Autodesk Inventor part; units mm, degrees
ref_plane "YZ Plane" through (0, 0, 0) normal (1, 0, 0) x (0, 1, 0)
ref_plane "XZ Plane" through (0, 0, 0) normal (0, 1, 0) x (-1, 0, 0)
ref_plane "XY Plane" through (0, 0, 0) normal (0, 0, 1) x (1, 0, 0)
sketch "Sketch1" plane through (0, 0, 0) normal (0, 0, 1) x (1, 0, 0)
  line L0 (-45, -34) -> (45, -34)
  line L1 (52, -27) -> (52, 27)
  line L2 (45, 34) -> (-45, 34)
  line L3 (-52, 27) -> (-52, -27)
  line L4 (-52, -34) -> (52, 34) construction
  line L5 (52, -34) -> (-52, 34) construction
  line L6 (-45, 27) -> (45, 27) construction
  line L7 (45, 27) -> (45, -27) construction
  line L8 (45, -27) -> (-45, -27) construction
  line L9 (-45, -27) -> (-45, 27) construction
  arc A0 (-45, 34) -> (-52, 27) centre (-45, 27) ccw
  arc A1 (52, 27) -> (45, 34) centre (45, 27) ccw
  arc A2 (45, -34) -> (52, -27) centre (45, -27) ccw
  arc A3 (-52, -27) -> (-45, -34) centre (-45, -27) ccw
  point P0 (0, 0)
  dimension "d0" = 104
  dimension "d1" = 68
  dimension "d2" = 54
  dimension "d3" = 90
extrude "Extrusion1" add sketch "Sketch1" along normal mid plane 4
sketch "Sketch2" plane through (0, 0, 2) normal (0, 0, 1) x (1, 0, 0)
  line L0 (45, 34) -> (-45, 34)
  arc A0 (-45, 34) -> (-52, 27) centre (-45, 27) ccw
  line L1 (-52, 27) -> (-52, -27)
  arc A1 (-52, -27) -> (-45, -34) centre (-45, -27) ccw
  line L2 (-45, -34) -> (45, -34)
  arc A2 (45, -34) -> (52, -27) centre (45, -27) ccw
  line L3 (52, -27) -> (52, 27)
  arc A3 (52, 27) -> (45, 34) centre (45, 27) ccw
  circle A4 centre (-45, 27) radius 2.75
  circle A5 centre (45, 27) radius 2.75
  circle A6 centre (45, -27) radius 2.75
  circle A7 centre (-45, -27) radius 2.75
  point P0 (0, 0)
  dimension "d7" = 5.5
extrude "Extrusion2" add sketch "Sketch2" along normal blind 5.3 contours A4 | A5 | A6 | A7
sketch "Sketch3" plane through (0, 0, -2) normal (0, 0, -1) x (-1, 0, 0)
  line L0 (45, 34) -> (-45, 34)
  arc A0 (-45, 34) -> (-52, 27) centre (-45, 27) ccw
  line L1 (-52, 27) -> (-52, -27)
  arc A1 (-52, -27) -> (-45, -34) centre (-45, -27) ccw
  line L2 (-45, -34) -> (45, -34)
  arc A2 (45, -34) -> (52, -27) centre (45, -27) ccw
  line L3 (52, -27) -> (52, 27)
  arc A3 (52, 27) -> (45, 34) centre (45, 27) ccw
  circle A4 centre (-45, 27) radius 2.75
  point P0 (0, 0)
hole "Hole1" at (-45, -27, -2) at (45, -27, -2) at (45, 27, -2) at (-45, 27, -2) direction (0, 0, 1) diameter 2.642 end through all
sketch "Sketch4" plane through (0, 0, 2) normal (0, 0, 1) x (1, 0, 0)
  line L0 (-12.5, -12.5) -> (12.5, -12.5)
  line L1 (12.5, -12.5) -> (12.5, 12.5)
  line L2 (12.5, 12.5) -> (-12.5, 12.5)
  line L3 (-12.5, 12.5) -> (-12.5, -12.5)
  line L4 (-12.5, -12.5) -> (12.5, 12.5) construction
  line L5 (12.5, -12.5) -> (-12.5, 12.5) construction
  point P0 (0, 0)
  dimension "d17" = 25
extrude "Extrusion3" cut sketch "Sketch4" against normal blind 3.35
properties part number "BackBracket" material "Steel, Mild"
Can you work these out from the model? Positions are in its coordinate system, mm. A direction names the side the tool comes from. Round coordinates to 2 decimals unless told otherwise and drop trailing zeros. Write each loop counter-clockwise with the first axis right and the second up, starting at its lowest first coordinate (ties: lowest second). Pieces come first, ordered by that corner, then holes. Notation, with made-up numbers: M -35,-16.75 L 2,-16.75 A15 ccw 2,-3.75 Z; hole C -21,80.25 d9. An arc over 180 degrees is marked long. Use a Markdown table: item, result.
Item 1: For pin 1 Ø20.5 at (x, y) = (-4.5, -4.5) entering from +Z; pin 2 Ø4 at (x, y) = (-45, -27) entering from +Z; pin 3 Ø5 at (y, z) = (-24.5, 6) entering from +X; pin 4 Ø5 at (x, z) = (40, 5.5) entering from +Y, each with a flat end and sliding along its axis, tell me the tip position at first contact or that it passes through.
Found:
| item | result |
|---|---|
| pin 1 | stops at z = 2 |
| pin 2 | stops at z = 7.3 |
| pin 3 | stops at x = 47.75 |
| pin 4 | stops at y = 28.15 |
Item 2: I want a section at A-A (y = -4.5). List the corners of the cut face in (x, z) for me, and give its area (3 significant figures).
Found:
| item | result |
|---|---|
| outline | M -52,-2 L 52,-2 L 52,2 L 12.5,2 L 12.5,-1.35 L -12.5,-1.35 L -12.5,2 L -52,2 Z |
| area | 332 mm2 |
Item 3: I want a section at C-C (x = 25.5). List the corners of the cut face in (y, z) for me.
Found:
| item | result |
|---|---|
| outline | M -34,-2 L 34,-2 L 34,2 L -34,2 Z |
Item 4: I want a section at B-B (x = -8). List the corners of the cut face in (y, z) for me, and give its area (3 significant figures).
Found:
| item | result |
|---|---|
| outline | M -34,-2 L 34,-2 L 34,2 L 12.5,2 L 12.5,-1.35 L -12.5,-1.35 L -12.5,2 L -34,2 Z |
| area | 188 mm2 |
Item 5: Which directions (+Z, -Z, +X, -X, +Y, -Y) give clear straight access to the entire face, cutting with the end or side of a thin tool? Please do faces 1 (the face through (12.5, 0, 0)), 2 (the face through (46.17, -26.39, 2.72)).
Found:
| item | result |
|---|---|
| face 1 | +Z |
| face 2 | +Z, -Z |
Item 6: I want a section at D-D (y = 14). List the corners of the cut face in (x, z) for me.
Found:
| item | result |
|---|---|
| outline | M -52,-2 L 52,-2 L 52,2 L -52,2 Z |
Item 7: If I drill on line 1 along X through (y, z) = (2.5, -1.25); line 2 along X through (y, z) = (-27, 1.5); line 3 along X through (y, z) = (-26, 1.75), over which ranges is the centre line in solid material (lowest first)? Write a range as [from, to].
Found:
| item | result |
|---|---|
| line 1 | x = [-52, -12.5], [12.5, 52] |
| line 2 | x = [-52, -46.32], [-43.68, 43.68], [46.32, 52] |
| line 3 | x = [-52, -45.86], [-44.14, 44.14], [45.86, 52] |
Item 8: We'd pull the mould along X, two halves only. Please class faces 3 (the face through (1, 34, 0)), 4 (the face through (49.9, 32, 0)), 5 (the face through (0, -12.5, 0)): released by +X, released by -X, zero draft, split by the parting line, or undercut.
Found:
| item | result |
|---|---|
| face 3 | zero draft |
| face 4 | released by +X |
| face 5 | undercut |
